```python
from build123d import *

# Parameters (mm, degrees)
SKETCH2_R      = 8.001
EXTRUDE2_DEPTH = 8.382
CHAMFER1_SIZE  = 1.016
EXTRUDE3_REACH = 10.382
SKETCH1_R      = 4.7625


with BuildPart() as part:
    # Sketch2 → Extrude2 (new body)
    with BuildSketch(Plane(origin=(0, 0, 0), x_dir=(1, 0, 0), z_dir=(0, 1, 0))):
        Circle(SKETCH2_R)
    extrude(amount=EXTRUDE2_DEPTH)

    # Chamfer1
    chamfer1_edges = [part.edges().sort_by_distance(p)[0] for p in [
        (-8.001, 0, 0),
        (-8.001, 8.382, 0),
    ]]
    chamfer(chamfer1_edges, length=CHAMFER1_SIZE)

    # Sketch1 → Extrude3 (cut, up to next)
    with BuildSketch(Plane(origin=(0, 0, 0), x_dir=(1, 0, 0), z_dir=(0, 1, 0)), mode=Mode.PRIVATE) as extrude3_sk1:
        with BuildLine():
            ThreePointArc((-8.138906745, 0), (-7.0485, -4.069453372), (-4.069453372, -7.0485))
            Line((-4.069453372, -7.0485), (-8.138906745, 0))
        make_face()
    extrude3_tool1 = extrude(extrude3_sk1.sketch, amount=EXTRUDE3_REACH, mode=Mode.PRIVATE) & part.part
    add(extrude3_tool1.solids().sort_by_distance((-6.484164, 0, 3.743634))[0], mode=Mode.SUBTRACT)
    # Sketch1 → Extrude3 (cut, up to next)
    with BuildSketch(Plane(origin=(0, 0, 0), x_dir=(1, 0, 0), z_dir=(0, 1, 0)), mode=Mode.PRIVATE) as extrude3_sk2:
        with BuildLine():
            ThreePointArc((-4.069453372, 7.0485), (-7.0485, 4.069453372), (-8.138906745, 0))
            Line((-8.138906745, 0), (-4.069453372, 7.0485))
        make_face()
    extrude3_tool2 = extrude(extrude3_sk2.sketch, amount=EXTRUDE3_REACH, mode=Mode.PRIVATE) & part.part
    add(extrude3_tool2.solids().sort_by_distance((-6.484164, 0, -3.743634))[0], mode=Mode.SUBTRACT)
    # Sketch1 → Extrude3 (cut, up to next)
    with BuildSketch(Plane(origin=(0, 0, 0), x_dir=(1, 0, 0), z_dir=(0, 1, 0)), mode=Mode.PRIVATE) as extrude3_sk3:
        Circle(SKETCH1_R)
    extrude3_tool3 = extrude(extrude3_sk3.sketch, amount=EXTRUDE3_REACH, mode=Mode.PRIVATE) & part.part
    add(extrude3_tool3.solids().sort_by_distance((0, 0, 0))[0], mode=Mode.SUBTRACT)
    # Sketch1 → Extrude3 (cut, up to next)
    with BuildSketch(Plane(origin=(0, 0, 0), x_dir=(1, 0, 0), z_dir=(0, 1, 0)), mode=Mode.PRIVATE) as extrude3_sk4:
        with BuildLine():
            Line((-4.069453372, 7.0485), (4.069453372, 7.0485))
            ThreePointArc((4.069453372, 7.0485), (0, 8.138906745), (-4.069453372, 7.0485))
        make_face()
    extrude3_tool4 = extrude(extrude3_sk4.sketch, amount=EXTRUDE3_REACH, mode=Mode.PRIVATE) & part.part
    add(extrude3_tool4.solids().sort_by_distance((0, 0, -7.487268))[0], mode=Mode.SUBTRACT)
    # Sketch1 → Extrude3 (cut, up to next)
    with BuildSketch(Plane(origin=(0, 0, 0), x_dir=(1, 0, 0), z_dir=(0, 1, 0)), mode=Mode.PRIVATE) as extrude3_sk5:
        with BuildLine():
            Line((4.069453372, 7.0485), (8.138906745, 0))
            ThreePointArc((8.138906745, 0), (7.0485, 4.069453372), (4.069453372, 7.0485))
        make_face()
    extrude3_tool5 = extrude(extrude3_sk5.sketch, amount=EXTRUDE3_REACH, mode=Mode.PRIVATE) & part.part
    add(extrude3_tool5.solids().sort_by_distance((6.484164, 0, -3.743634))[0], mode=Mode.SUBTRACT)
    # Sketch1 → Extrude3 (cut, up to next)
    with BuildSketch(Plane(origin=(0, 0, 0), x_dir=(1, 0, 0), z_dir=(0, 1, 0)), mode=Mode.PRIVATE) as extrude3_sk6:
        with BuildLine():
            Line((8.138906745, 0), (4.069453372, -7.0485))
            ThreePointArc((4.069453372, -7.0485), (7.0485, -4.069453372), (8.138906745, 0))
        make_face()
    extrude3_tool6 = extrude(extrude3_sk6.sketch, amount=EXTRUDE3_REACH, mode=Mode.PRIVATE) & part.part
    add(extrude3_tool6.solids().sort_by_distance((6.484164, 0, 3.743634))[0], mode=Mode.SUBTRACT)
    # Sketch1 → Extrude3 (cut, up to next)
    with BuildSketch(Plane(origin=(0, 0, 0), x_dir=(1, 0, 0), z_dir=(0, 1, 0)), mode=Mode.PRIVATE) as extrude3_sk7:
        with BuildLine():
            ThreePointArc((-4.069453372, -7.0485), (0, -8.138906745), (4.069453372, -7.0485))
            Line((4.069453372, -7.0485), (-4.069453372, -7.0485))
        make_face()
    extrude3_tool7 = extrude(extrude3_sk7.sketch, amount=EXTRUDE3_REACH, mode=Mode.PRIVATE) & part.part
    add(extrude3_tool7.solids().sort_by_distance((0, 0, 7.487268))[0], mode=Mode.SUBTRACT)


solid = part.part
```
Check sheet for the modelled part. Datum: model origin and axes. Units: mm. Coordinates: 2 decimals unless noted, no trailing zeros. Write each loop counter-clockwise with the first axis right and the second up, starting at its lowest first coordinate (ties: lowest second). Pieces come first, ordered by that corner, then holes. Notation, with made-up numbers: M 47.5,-14 L 99.5,-14 A21 cw 99.5,14 Z; hole C -8,7 d10. An arc over 180 degrees is marked long. Write item = value, one per line. Start each with the question number.
1. Sectioned sample at B-B (y = 1.5). Record the cut outline in (x, z) (1 decimal), then the cut area to 3 significant figures.
2. Sectioned sample at C-C (z = 0). Record the cut outline in (x, y) (1 decimal).
3. Thickness scan on probe 1 along X at (y, z) = (6.5, 0); probe 2 along Z at (x, y) = (0, 4); probe 3 along Z at (x, y) = (1.75, 6.25). Record the ranges inside material, lowest first.
4. Go/stop test with flat-tipped pins: pin 1 (4 mm diameter, centred on y = 3, z = -4.5, fed in from -X); pin 2 (6 mm diameter, centred on x = -1, z = -0.5, fed in from -Y). Record where each tip stops, or that it passes through.
5. Mould release check, pull along Z, two halves, no side actions. Record for faces 1 (the cylindrical face through (-3.78, 4.13, 2.9)), 2 (the flat face through (6.13, 4.13, 3.48)), 3 (the flat face through (-6.13, 4.13, -3.48)): pulls with the +Z half, pulls with the -Z half, needs draft (parallel to the pull), parting line crosses it, or undercut.
The answers:
q1.outline = M -8,-0.2 L -4.2,-6.8 A8 ccw -3.8,-7 L 3.8,-7 A8 ccw 4.2,-6.8 L 8,-0.2 A8 ccw 8,0.2 L 4.2,6.8 A8 ccw 3.8,7 L -3.8,7 A8 ccw -4.2,6.8 L -8,0.2 A8 ccw Z; hole C 0,0 d9.5
q1.area = 101 mm²
q2.outline = M -8,1 L -7,0 L -4.8,0 L -4.8,8.4 L -7,8.4 L -8,7.4 Z; M 4.8,0 L 7,0 L 8,1 L 8,7.4 L 7,8.4 L 4.8,8.4 Z
q3.probe_1 = -8 to -4.76, 4.76 to 8
q3.probe_2 = -7.05 to -4.76, 4.76 to 7.05
q3.probe_3 = -7.05 to -4.43, 4.43 to 7.05
q4.pin_1 = -6.7
q4.pin_2 = through
q5.face_1 = undercut
q5.face_2 = pulls with the +Z half
q5.face_3 = pulls with the -Z half
